```python
from build123d import *

# Parameters (mm, degrees)
SKETCH1_R           = 15
BOSS_EXTRUDE1_DEPTH = 3
SKETCH2_R           = 2.75
CUT_EXTRUDE1_DEPTH  = 11
SKETCH3_R           = 1.7
CUT_EXTRUDE5_DEPTH  = 10
CIRPATTERN1_COUNT   = 13
CUT_EXTRUDE6_DEPTH  = 10
CIRPATTERN2_COUNT   = 13


with BuildPart() as part:
    # Sketch1 → Boss-Extrude1 (new body)
    with BuildSketch(Plane.XY):
        Circle(SKETCH1_R)
    extrude(amount=BOSS_EXTRUDE1_DEPTH)

    # Sketch2 → Cut-Extrude1 (cut)
    with BuildSketch(Plane.XY.offset(3)):
        Circle(SKETCH2_R)
    extrude(amount=-CUT_EXTRUDE1_DEPTH, mode=Mode.SUBTRACT)

    # Sketch3 → Cut-Extrude5 (cut)
    with BuildSketch(Plane.XY.offset(3)):
        with Locations((3.738719386, 12.815790157)):
            Circle(SKETCH3_R)
    cut_extrude5 = extrude(amount=-CUT_EXTRUDE5_DEPTH, mode=Mode.SUBTRACT)

    # CirPattern1: Cut-Extrude5 ×13 about axis
    cirpattern1_axis = Axis((0, 0, 0), (0, 0, 1))
    for i in range(1, CIRPATTERN1_COUNT):
        add(cut_extrude5.rotate(cirpattern1_axis, i * 360 / CIRPATTERN1_COUNT), mode=Mode.SUBTRACT)

    # Sketch4 → Cut-Extrude6 (cut)
    with BuildSketch(Plane.XY.offset(3)):
        Polygon((-1.22331177, 12.153685267), (0.632651304, 14.986652472), (2.243253238, 12.007346591), (4.816692291, 13.980883612), (-0.349444611, 17.339445828), (-3.866613741, 14.072309299), align=None)
    cut_extrude6 = extrude(amount=-CUT_EXTRUDE6_DEPTH, mode=Mode.SUBTRACT)

    # CirPattern2: Cut-Extrude6 ×13 about axis
    cirpattern2_axis = Axis((0, 0, 0), (0, 0, 1))
    for i in range(1, CIRPATTERN2_COUNT):
        add(cut_extrude6.rotate(cirpattern2_axis, i * 360 / CIRPATTERN2_COUNT), mode=Mode.SUBTRACT)


solid = part.part
```
Model file for the job. Use its own axes, mm. A direction names the side the tool comes from. Coordinates: 2 decimals unless noted, no trailing zeros. Write each loop counter-clockwise with the first axis right and the second up, starting at its lowest first coordinate (ties: lowest second). Pieces come first, ordered by that corner, then holes. Notation, with made-up numbers: (-37.75, 63.5) - (-13.75, 63.5) arc R24 cw to (-13.75, 92.5) - close; hole circle Ø6 at (-36.5, 89). An arc over 180 degrees is marked (long way). Use a Markdown table: item, result. Add a question column.
Item 1: Band-saw the part on A-A, the plane x = 0. Write the cut outline in (y, z).
Item 2: 3-axis set-ups, long thin cutter, end or side, ignore diameter. For faces 4 (the face through (-8.755, -10.347, 1.521)), 5 (the face through (0, -3, 3)), 6 (the face through (1.427, 13.518, 1.521)), 7 (the face through (-13.49, 1.33, 1.52)): which of +Z, -Z, +X, -X, +Y, -Y reach the whole face in a straight line?
Item 3: Drop flat-ended pins along their axis: pin 1 (1.5 mm diameter, centred on x = 7, z = 0.5, fed in from -Y); pin 2 (1 mm diameter, centred on y = -9.5, z = 0.5, fed in from +X); pin 3 (10 mm diameter, centred on x = 11, y = 9, fed in from -Z); pin 4 (4.5 mm diameter, centred on x = 0, y = 0, fed in from +Z). Give the stop position or say it passes through.
Item 4: Drill centre lines: line 1 along X through (y, z) = (12, 0.95); line 2 along Y through (x, z) = (0, 0.8); line 3 along X through (y, z) = (-12.5, 2.75). Where is each one in solid material? Low to high.
Item 5: Band-saw the part on C-C, the plane y = -8.75. Write the cut outline in (x, z).
Item 6: Band-saw the part on B-B, the plane x = 13.25. Write the cut outline in (y, z), and give its area (3 significant figures).
Item 7: Two-plate mould, pull along X, no slides. Class faces 1 (the face through (13.59, 0.21, 1.52)), 2 (the face through (-2.943, -13.23, 1.521)), 3 (the face through (-11.327, 7.444, 1.521)): pulls with the +X half, pulls with the -X half, needs draft (parallel to the pull), parting line crosses it, or undercut.
A:
| question | item | result |
|---|---|---|
| 1 | outline | (-11.73, 0) - (-2.75, 0) - (-2.75, 3) - (-11.73, 3) - close; (2.75, 0) - (14.02, 0) - (14.02, 3) - (2.75, 3) - close |
| 2 | face 4 | +Z, -Z, -Y |
| 2 | face 5 | +Z, +X, -X, +Y, -Y |
| 2 | face 6 | +Z, -Z, +Y |
| 2 | face 7 | +Z, -Z, -X |
| 3 | pin 1 | stops at y = -11.01 |
| 3 | pin 2 | stops at x = 9.23 |
| 3 | pin 3 | stops at z = 0 |
| 3 | pin 4 | passes through |
| 4 | line 1 | x = -6.56 to -4.08, -1.34 to 2.25, 5.77 to 7.54 |
| 4 | line 2 | y = -11.73 to -2.75, 2.75 to 14.02 |
| 4 | line 3 | x = -4.69 to -2.16, 0.97 to 3.75 |
| 5 | outline | (-9.93, 0) - (9.04, 0) - (9.04, 3) - (-9.93, 3) - close |
| 6 | outline | (-5.98, 0) - (-5.16, 0) - (-5.16, 3) - (-5.98, 3) - close; (-0.03, 0) - (2.02, 0) - (2.02, 3) - (-0.03, 3) - close |
| 6 | area | 8.59 mm² |
| 7 | face 1 | pulls with the +X half |
| 7 | face 2 | undercut |
| 7 | face 3 | pulls with the -X half |
